Read the model definition and answer for the solid it produces. Units are mm, in the model's axes. A direction names the side the tool comes from. Coordinates: 2 decimals unless noted, no trailing zeros. Loops run counter-clockwise (first coordinate to the right, second up) from the corner with the lowest first, then second, coordinate; pieces in that order, holes last.
from build123d import *

# Parameters (mm, degrees)
SKETCH1_W           = 250
SKETCH1_H           = 33.2
BOSS_EXTRUDE1_DEPTH = 1.6
SKETCH2_R           = 5
CUT_EXTRUDE1_DEPTH  = 127.107573127


with BuildPart() as part:
    # Sketch1 → Boss-Extrude1 (new body)
    with BuildSketch(Plane(origin=(0, 0, 0), x_dir=(1, 0, 0), z_dir=(0, 1, 0))):
        Rectangle(SKETCH1_W, SKETCH1_H)
    extrude(amount=-BOSS_EXTRUDE1_DEPTH)

    # Sketch2 → Cut-Extrude1 (cut, through all)
    with BuildSketch(Plane(origin=(0, 0, 0), x_dir=(1, 0, 0), z_dir=(0, 1, 0))):
        with Locations(Location((-38.8, 0, 0), (0, 0, 270))):
            Circle(SKETCH2_R)
        with Locations(Location((-0.8, 0, 0), (0, 0, 270))):
            Circle(SKETCH2_R)
        with BuildLine():
            Line((-108.4, 15), (-70.4, 15))
            ThreePointArc((-70.4, 15), (-55.4, 0), (-70.4, -15))
            Line((-70.4, -15), (-108.4, -15))
            ThreePointArc((-108.4, -15), (-123.4, 0), (-108.4, 15))
        make_face()
    extrude(amount=-CUT_EXTRUDE1_DEPTH, mode=Mode.SUBTRACT)


solid = part.part
Item 1: A cutting plane is placed at B-B on y = -0.75. Determine the outline of the cut face in (x, z), then the cut area to 3 significant figures.
Numbers:
outline: (-125, -16.6) - (125, -16.6) - (125, 16.6) - (-125, 16.6) - close; hole (-108.4, -15) - (-70.4, -15) arc R15 ccw to (-70.4, 15) - (-108.4, 15) arc R15 ccw to start; hole circle Ø10 at (-38.8, 0); hole circle Ø10 at (-0.8, 0)
area: 6,300 mm2
Item 2: A cutting plane is placed at C-C on z = 9.5. Determine the outline of the cut face in (x, y), then the cut area to 3 significant figures.
Numbers:
outline: (-125, -1.6) - (-120.01, -1.6) - (-120.01, 0) - (-125, 0) - close; (-58.79, -1.6) - (125, -1.6) - (125, 0) - (-58.79, 0) - close
area: 302 mm2
Item 3: A cutting plane is placed at A-A on x = -83. Determine the outline of the cut face in (y, z), then the cut area to 3 significant figures.
Numbers:
outline: (-1.6, -16.6) - (0, -16.6) - (0, -15) - (-1.6, -15) - close; (-1.6, 15) - (0, 15) - (0, 16.6) - (-1.6, 16.6) - close
area: 5.12 mm2
Item 4: Given pin 1 (8 mm diameter, centred on x = -0.8, z = 0, fed in from +Y), flat-ended and moving along its own axis, determine where the tip first touches the part or whether it passes through.
Numbers:
pin 1: passes through
Item 5: Which of the six approach directions +Z, -Z, +X, -X, +Y, -Y give full straight-line access (tool end or side, diameter ignored) to faces 3 (the face through (26, 0, 0)), 4 (the face through (-55.404, -0.789, -0.33))?
Numbers:
face 3: +Z, -Z, +X, -X, +Y
face 4: +Y, -Y
Item 6: Find the intervals of material crossed by line 1 along X through (y, z) = (-0.6, 0); line 2 along X through (y, z) = (-0.4, 3); line 3 along Z through (x, y) = (-98, -0.4), in increasing order.
Numbers:
line 1: x = -125 to -123.4, -55.4 to -43.8, -33.8 to -5.8, 4.2 to 125
line 2: x = -125 to -123.1, -55.7 to -42.8, -34.8 to -4.8, 3.2 to 125
line 3: z = -16.6 to -15, 15 to 16.6
Item 7: Determine the mould class of faces 1 (the face through (-5.68, -0.79, -1.08)), 2 (the face through (26, -1.6, 0)) for opening direction Z: released by +Z, released by -Z, zero draft, split by the parting line, or undercut.
Numbers:
face 1: undercut
face 2: zero draft
